Geometry check sheet. Reference: the model listing, model coordinates, mm. Face numbers are marked on the shaded views. Give positions to 0.01 mm unless a question says otherwise; leave off trailing zeros. Loops run counter-clockwise (first coordinate to the right, second up) from the corner with the lowest first, then second, coordinate; pieces in that order, holes last.
1. Cross-section at D-D, the plane z = -1.5. Record the cut outline in (x, y), plus the area to 3 significant figures.
2. Cross-section at C-C, the plane x = 11.5. Record the cut outline in (y, z).
3. Go/stop test with flat-tipped pins: pin 1 Ø2.5 at (x, z) = (5.5, 13) entering from +Y; pin 2 Ø1.7 at (x, z) = (5.5, 18) entering from +Y; pin 3 Ø9.5 at (x, z) = (6.34, 9.46) entering from +Y; pin 4 Ø0.6 at (x, y) = (6, -0.5) entering from +Z. Record where each tip stops, or that it passes through.
4. Material ranges on L1, parallel to X at y = 0.5, z = 21.5; L2, parallel to Z at x = 1.5, y = -1.2; L3, parallel to X at y = -0.9, z = 4, recorded low to high.
5. Cross-section at B-B, the plane y = -1.1. Record the cut outline in (x, z), plus the area to 3 significant figures.
6. Release check for a two-part mould opening along X. For the marked faces 1 and 2 record: +X half, -X half, draft (parallel to the pull), parting line (faces both ways), or undercut.
7. Cross-section at A-A, the plane z = 23. Record the cut outline in (x, y).
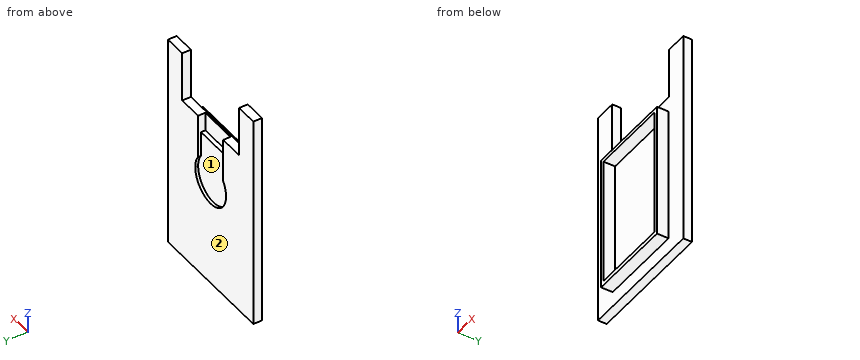
from build123d import *

# Parameters (mm, degrees)
SKETCH1_W           = 22.86
SKETCH1_H           = 38.1
BOSS_EXTRUDE1_DEPTH = 1.524
SKETCH2_W           = 14.986
SKETCH2_H           = 23.876
SKETCH2_W_2         = 13.716
SKETCH2_H_2         = 22.479
BOSS_EXTRUDE2_DEPTH = 2.032
CUT_EXTRUDE2_DEPTH  = 0.508
CUT_EXTRUDE3_START  = 0.508
SKETCH6_W           = 15.24
SKETCH6_H           = 8.89
CUT_EXTRUDE3_DEPTH  = 35.245345025
SKETCH7_W           = 6.731
SKETCH7_H           = 3.302
CUT_EXTRUDE4_DEPTH  = 0.762


with BuildPart() as part:
    # Sketch1 → Boss-Extrude1 (new body)
    with BuildSketch(Plane(origin=(0, 0, 0), x_dir=(1, 0, 0), z_dir=(0, 1, 0))):
        with Locations((6.342648046, -9.464051393)):
            Rectangle(SKETCH1_W, SKETCH1_H)
    extrude(amount=BOSS_EXTRUDE1_DEPTH)

    # Sketch2 → Boss-Extrude2 (add)
    with BuildSketch(Plane.XZ):
        with Locations((6.342648046, 5.019051393)):
            Rectangle(SKETCH2_W, SKETCH2_H)
        with Locations((6.342648046, 5.082551393)):
            Rectangle(SKETCH2_W_2, SKETCH2_H_2, mode=Mode.SUBTRACT)
    extrude(amount=BOSS_EXTRUDE2_DEPTH)

    # Sketch5 → Cut-Extrude2 (cut)
    with BuildSketch(Plane(origin=(0, 1.524, 0), x_dir=(1, 0, 0), z_dir=(0, 1, 0))):
        with BuildLine():
            ThreePointArc((10.470148046, -9.464051393), (5.088623524, -5.531662964), (2.977148046, -11.853542133))
            Line((2.977148046, -11.853542133), (9.708148046, -11.853542133))
            ThreePointArc((9.708148046, -11.853542133), (10.275036474, -10.718075914), (10.470148046, -9.464051393))
        make_face()
        with BuildLine():
            Line((9.708148046, -11.853542133), (2.977148046, -11.853542133))
            ThreePointArc((2.977148046, -11.853542133), (6.342648046, -13.591551393), (9.708148046, -11.853542133))
        make_face()
        with BuildLine():
            ThreePointArc((9.708148046, -11.853542133), (6.342648046, -13.591551393), (2.977148046, -11.853542133))
            Line((2.977148046, -11.853542133), (2.977148046, -28.514051393))
            Line((2.977148046, -28.514051393), (9.708148046, -28.514051393))
            Line((9.708148046, -28.514051393), (9.708148046, -11.853542133))
        make_face()
    extrude(amount=-CUT_EXTRUDE2_DEPTH, mode=Mode.SUBTRACT)

    # Sketch6 → Cut-Extrude3 (cut, through all)
    with BuildSketch(Plane(origin=(0, 1.016, 0), x_dir=(1, 0, 0), z_dir=(0, 1, 0)).offset(CUT_EXTRUDE3_START)):
        with Locations((6.342648046, -24.069051393)):
            Rectangle(SKETCH6_W, SKETCH6_H)
    extrude(amount=-CUT_EXTRUDE3_DEPTH, mode=Mode.SUBTRACT)

    # Sketch7 → Cut-Extrude4 (cut)
    with BuildSketch(Plane(origin=(0, 1.016, 0), x_dir=(1, 0, 0), z_dir=(0, 1, 0))):
        with Locations((6.342648046, -17.973051393)):
            Rectangle(SKETCH7_W, SKETCH7_H)
    extrude(amount=-CUT_EXTRUDE4_DEPTH, mode=Mode.SUBTRACT)


solid = part.part
Result:
1. outline: (-5.09, 0) - (-1.15, 0) - (-1.15, -2.03) - (-0.52, -2.03) - (-0.52, 0) - (13.2, 0) - (13.2, -2.03) - (13.84, -2.03) - (13.84, 0) - (17.77, 0) - (17.77, 1.52) - (-5.09, 1.52) - close
1. area: 37.4 mm2
2. outline: (-2.03, -6.92) - (0, -6.92) - (0, -9.59) - (1.52, -9.59) - (1.52, 19.62) - (0, 19.62) - (0, 16.96) - (-2.03, 16.96) - (-2.03, 16.32) - (0, 16.32) - (0, -6.16) - (-2.03, -6.16) - close
3. pin 1: stops at y = 1.02
3. pin 2: stops at y = 0.25
3. pin 3: stops at y = 1.52
3. pin 4: stops at z = 16.96
4. L1: x = -5.09 to -1.28, 13.96 to 17.77
4. L2: z = -6.92 to -6.16, 16.32 to 16.96
4. L3: x = -1.15 to -0.52, 13.2 to 13.84
5. outline: (-1.15, -6.92) - (13.84, -6.92) - (13.84, 16.96) - (-1.15, 16.96) - close; hole (-0.52, -6.16) - (13.2, -6.16) - (13.2, 16.32) - (-0.52, 16.32) - close
5. area: 49.5 mm2
6. face 1: undercut
6. face 2: draft
7. outline: (-5.09, 0) - (-1.28, 0) - (-1.28, 1.52) - (-5.09, 1.52) - close; (13.96, 0) - (17.77, 0) - (17.77, 1.52) - (13.96, 1.52) - close
